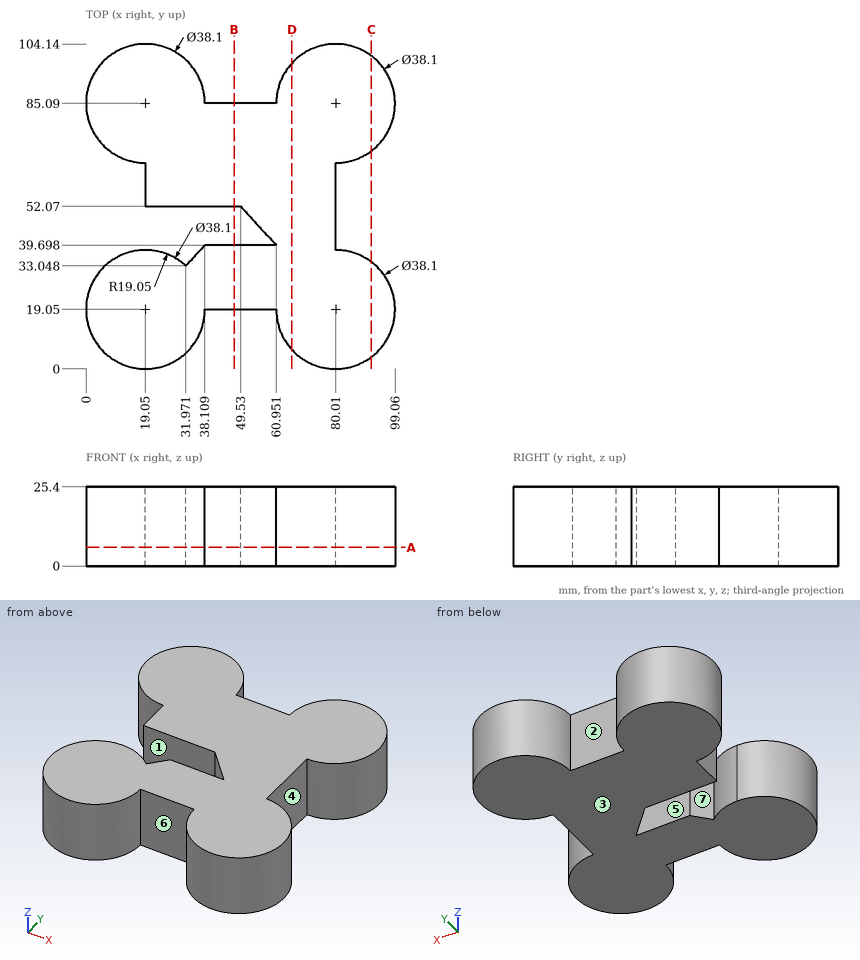
Design review of the part shown in the three views and the two pictorial views. Dimensions are in mm from the part's minimum x, y and z. A direction names the side the tool comes from. Give positions to 0.01 mm unless a question says otherwise; leave off trailing zeros. Loops run counter-clockwise (first coordinate to the right, second up) from the corner with the lowest first, then second, coordinate; pieces in that order, holes last. Notation, with made-up numbers: (48.5, 64) - (105.5, 64) arc R13 cw to (105.5, 68) - close; hole circle Ø1 at (13, 67). An arc over 180 degrees is marked (long way). Answer as a JSON object with one key per item and string values.
Q1. For the marked faces 4, 5, 6 and 7, list the 3-axis set-ups (+Z, -Z, +X, -X, +Y, -Y) from which the entire face can be reached by the end or side of a thin tool; tool diameter is ignored.
Worked out:
{"face 4": "+Z, -Z, +X", "face 5": "+Z, -Z, -X", "face 6": "+Z, -Z, -Y", "face 7": "+Z, -Z"}
Q2. To check wall thickness, follow line 1 along Y through (x, z) = (19.5, 7) (1 decimal); line 2 along Y through (x, z) = (19, 3.75); line 3 along X through (y, z) = (18.5, 4.75). State the ranges of each line that lie inside material, in increasing order.
Worked out:
{"line 1": "y = 0 to 38.1, 52.1 to 104.1", "line 2": "y = 0 to 38.1, 66.04 to 104.14", "line 3": "x = 0.01 to 38.09, 60.97 to 99.05"}
Q3. Add section D-D on x = 66. State the section outline as (y, z) points.
Worked out:
{"outline": "(6.14, 0) - (98, 0) - (98, 25.4) - (6.14, 25.4) - close"}
Q4. Add section C-C on x = 91.5. State the section outline as (y, z) points (1 decimal), plus the area to 3 significant figures.
Worked out:
{"outline": "(3.9, 0) - (34.2, 0) - (34.2, 25.4) - (3.9, 25.4) - close; (69.9, 0) - (100.3, 0) - (100.3, 25.4) - (69.9, 25.4) - close", "area": "1,540 mm^2"}
Q5. Mouldability with a two-part tool opening along Y and no side actions: class the marked faces 1, 2 and 3 as +Y half, -Y half, draft (parallel to the pull), parting line (faces both ways), or undercut.
Worked out:
{"face 1": "undercut", "face 2": "+Y half", "face 3": "draft"}
Q6. Add section A-A on z = 6. State the section outline as (x, y) points, plus the area to 3 significant figures.
Worked out:
{"outline": "(19.05, 52.07) - (49.53, 52.07) - (60.95, 39.7) - (38.11, 39.7) - (31.97, 33.05) arc R19.05 ccw (long way) to (38.1, 19.05) - (60.96, 19.05) arc R19.05 ccw (long way) to (80.01, 38.1) - (80.01, 66.04) arc R19.05 ccw (long way) to (60.96, 85.09) - (38.1, 85.09) arc R19.05 ccw (long way) to (19.05, 66.04) - close", "area": "6,940 mm^2"}
Q7. Add section B-B on x = 47.5. State the section outline as (y, z) points, plus the area to 3 significant figures.
Worked out:
{"outline": "(19.05, 0) - (39.7, 0) - (39.7, 25.4) - (19.05, 25.4) - close; (52.07, 0) - (85.09, 0) - (85.09, 25.4) - (52.07, 25.4) - close", "area": "1,360 mm^2"}
Q8. Insertion check: pin 1 (8 mm diameter, centred on y = 88.5, z = 9.5, fed in from +X); pin 2 (1 mm diameter, centred on y = 56, z = 14.5, fed in from +X); pin 3 (5 mm diameter, centred on y = 28.5, z = 19.5, fed in from +X); pin 4 (4 mm diameter, centred on y = 58.5, z = 13.5, fed in from -X). Each pin has a flat end and moves straight along its axis. Give the tip position at first contact, or say it passes through.
Worked out:
{"pin 1": "stops at x = 99.06", "pin 2": "stops at x = 80.01", "pin 3": "stops at x = 97.75", "pin 4": "stops at x = 19.05"}
